Check sheet for the modelled part. Datum: model origin and axes. Units: mm. A direction names the side the tool comes from. Round coordinates to 2 decimals unless told otherwise and drop trailing zeros. Write each loop counter-clockwise with the first axis right and the second up, starting at its lowest first coordinate (ties: lowest second). Pieces come first, ordered by that corner, then holes. Notation, with made-up numbers: (5, 85.5) - (17, 85.5) arc R18 cw to (17, 103.5) - close; hole circle Ø4 at (21, 88). An arc over 180 degrees is marked (long way). Use one line per item in the form item = value. Start each with the question number.
1) Section check D-D (x = 32.5). Record the boundary of the cut face in (y, z).
2) Set-up check for faces 4 (the face through (22.6, -16.41, 4.32)), 5 (the face through (31, -1.96, 12)), 6 (the face through (31, -3.085, 11)), 7 (the face through (25.19, 1.98, 0.99)), 8 (the face through (31, -19, 2)): record each of +Z, -Z, +X, -X, +Y, -Y from which the full face is reachable in a straight line by a thin tool's end or side.
3) Section check C-C (x = 23.75). Record the boundary of the cut face in (y, z).
4) Draft check along X on faces 1 (the face through (33.175, -21.45, 0.986)), 2 (the face through (31, -16.96, 12)), 3 (the face through (38, 1.9, 1)). Enter one of: +X half, -X half, draft (parallel to the pull), parting line (faces both ways), or undercut.
5) Gauge pin test, flat ends, axial feed: P1, Ø2, axis at x = 31.55, y = -21.96, coming from the -Z side; P2, Ø8, axis at x = 36, z = 11, coming from the +Y side; P3, Ø3.5, axis at x = 24.19, z = 5.53, coming from the -Y side; P4, Ø6.5, axis at x = 33.5, y = -10, coming from the +Z side. Record the tip position at first contact, or that the pin passes through.
6) Scan lines: probe 1 along X at (y, z) = (-10, 16.25); probe 2 along Y at (x, z) = (33.25, 6); probe 3 along Z at (x, y) = (40, -9). Record each from-to range of solid material in increasing order.
7) Section check A-A (z = 9). Record the boundary of the cut face in (x, y).
8) Section check B-B (y = 2.5). Record the boundary of the cut face in (x, z), then the cut area to 3 significant figures.
from build123d import *

# Parameters (mm, degrees)
F0_W     = 21
F0_H     = 15
F0_W_2   = 19.5
F0_H_2   = 12.75
F1_DEPTH = 22
F2_DEPTH = 1
F0_R     = 1.7
F3_DEPTH = 2
F4_R     = 3.4
F5_R     = 2
F6_DEPTH = 2.5


with BuildPart() as f1:
    # F0 (on Top) → F1 (new body)
    with BuildSketch(Plane.XY):
        with Locations((31.553322, -9.46031)):
            Rectangle(F0_W, F0_H)
        with Locations((31.553322, -9.46031)):
            Rectangle(F0_W_2, F0_H_2, mode=Mode.SUBTRACT)
    extrude(amount=F1_DEPTH)

    # F0 (on Top) → F2 (join)
    with BuildSketch(Plane.XY):
        with Locations((31.553322, -9.46031)):
            Rectangle(F0_W_2, F0_H_2)
    extrude(amount=F2_DEPTH)

    # F0 (on Top) → F3 (join)
    with BuildSketch(Plane.XY):
        Polygon((31.553322, 8.03969), (21.053322, -1.96031), (42.053322, -1.96031), align=None)
        with Locations((31.553322, 3.03969)):
            Circle(F0_R, mode=Mode.SUBTRACT)
        Polygon((42.053322, -16.96031), (21.053322, -16.96031), (31.553322, -26.96031), align=None)
        with Locations((31.553322, -21.96031)):
            Circle(F0_R, mode=Mode.SUBTRACT)
    extrude(amount=F3_DEPTH)

    # F4
    f4_edges = [f1.edges().sort_by_distance(p)[0] for p in [
        (31.553322, 8.03969, 1),
        (31.553322, -26.96031, 1),
    ]]
    fillet(f4_edges, radius=F4_R)

    # F5 (on face) → F6 (cut)
    with BuildSketch(Plane.XZ.offset(16.96031)):
        with Locations((24.191299, 5.534078)):
            Circle(F5_R)
    extrude(amount=-F6_DEPTH, mode=Mode.SUBTRACT)


solid = f1.part
Results are:
q1.outline = (-25.53, 0) - (-23.37, 0) - (-23.37, 2) - (-25.53, 2) - close; (-20.55, 0) - (1.63, 0) - (1.63, 2) - (-1.96, 2) - (-1.96, 22) - (-3.09, 22) - (-3.09, 1) - (-15.84, 1) - (-15.84, 22) - (-16.96, 22) - (-16.96, 2) - (-20.55, 2) - close; (4.45, 0) - (6.61, 0) - (6.61, 2) - (4.45, 2) - close
q2.face_4 = -Y
q2.face_5 = +Z, +X, -X, +Y
q2.face_6 = +Z
q2.face_7 = +Z, -Z, -X, +Y
q2.face_8 = +Z, +X, -X, -Y
q3.outline = (-19.53, 0) - (0.61, 0) - (0.61, 2) - (-1.96, 2) - (-1.96, 22) - (-3.09, 22) - (-3.09, 1) - (-15.84, 1) - (-15.84, 3.58) - (-16.96, 3.58) - (-16.96, 2) - (-19.53, 2) - close; (-16.96, 7.48) - (-15.84, 7.48) - (-15.84, 22) - (-16.96, 22) - close
q4.face_1 = undercut
q4.face_2 = draft
q4.face_3 = +X half
q5.P1 = through
q5.P2 = -1.96
q5.P3 = -3.09
q5.P4 = 1
q6.probe_1 = 21.05 to 21.8, 41.3 to 42.05
q6.probe_2 = -16.96 to -15.84, -3.09 to -1.96
q6.probe_3 = 0 to 1
q7.outline = (21.05, -16.96) - (42.05, -16.96) - (42.05, -1.96) - (21.05, -1.96) - close; hole (21.8, -15.84) - (41.3, -15.84) - (41.3, -3.09) - (21.8, -3.09) - close
q8.outline = (25.74, 0) - (29.94, 0) - (29.94, 2) - (25.74, 2) - close; (33.17, 0) - (37.37, 0) - (37.37, 2) - (33.17, 2) - close
q8.area = 16.8 mm²
